```python
from build123d import *

# Parameters (mm, degrees)
ESQUISSE1_R             = 1.6
BOSS_EXTRU_1_DEPTH      = 3
ENL_V_MAT_EXTRU_1_DEPTH = 10


with BuildPart() as part:
    # Esquisse1 → Boss.-Extru.1 (new body)
    with BuildSketch(Plane.XY):
        Polygon((-13.474992457, 0.072428093), (-16.723236211, 3.320852512), (-154.236345188, 3.320852512), (-157.478985875, 0.078211825), (-157.478985875, -70.04068474), (-131.779420125, -114.771472067), (-127.355917516, -115.9649154), (-106.081983802, -103.720194839), (-66.092540926, -97.775797545), (-55.98795635, -83.933633781), (-16.581747648, -83.933633781), (-13.474992457, -80.826878591), align=None)
        Polygon((-126.111124489, -102.556497988), (-140.02282508, -78.342807898), (-141.407217303, -75.981121034), (-120.346626934, -63.796065222), (-120.346308835, -12.429484403), (-101.345774335, -12.429484403), (-101.345774335, -9.929307079), (-82.344426674, -9.929307079), (-82.344426674, -7.679926158), (-62.343149943, -7.681038584), (-62.343149943, -9.929307079), (-43.477687779, -9.929307079), (-43.477687779, -14.679643994), (-24.474992457, -14.679643994), (-24.474992457, -72.933633781), (-61.577157206, -72.933633781), (-72.263087593, -87.572177036), (-109.761976756, -93.1463556), align=None, mode=Mode.SUBTRACT)
        with Locations((-68.897334865, -93.137788223)):
            Circle(ESQUISSE1_R, mode=Mode.SUBTRACT)
        with Locations((-146.02282508, -1.677868186)):
            Circle(ESQUISSE1_R, mode=Mode.SUBTRACT)
        with Locations((-18.474992457, -1.68453516)):
            Circle(ESQUISSE1_R, mode=Mode.SUBTRACT)
    extrude(amount=BOSS_EXTRU_1_DEPTH)

    # Esquisse2 → Enlèv. mat.-Extru.1 (cut)
    with BuildSketch(Plane.XY.offset(3)):
        with BuildLine():
            Line((-25.386559375, 6.054162745), (-25.386559375, -4.679147488))
            ThreePointArc((-25.386559375, -4.679147488), (-26.386559375, -5.679147488), (-27.386559375, -4.679147488))
            Line((-27.386559375, -4.679147488), (-27.386559375, 6.054162745))
            ThreePointArc((-27.386559375, 6.054162745), (-26.386559375, 7.054162745), (-25.386559375, 6.054162745))
        make_face()
        with BuildLine():
            Line((-29.386559375, 6.054162745), (-29.386559375, -4.679147488))
            ThreePointArc((-29.386559375, -4.679147488), (-30.386559375, -5.679147488), (-31.386559375, -4.679147488))
            Line((-31.386559375, -4.679147488), (-31.386559375, 6.054162745))
            ThreePointArc((-31.386559375, 6.054162745), (-30.386559375, 7.054162745), (-29.386559375, 6.054162745))
        make_face()
        with BuildLine():
            Line((-33.386559375, 6.054162745), (-33.386559375, -4.679147488))
            ThreePointArc((-33.386559375, -4.679147488), (-34.386559375, -5.679147488), (-35.386559375, -4.679147488))
            Line((-35.386559375, -4.679147488), (-35.386559375, 6.054162745))
            ThreePointArc((-35.386559375, 6.054162745), (-34.386559375, 7.054162745), (-33.386559375, 6.054162745))
        make_face()
        with BuildLine():
            Line((-37.386559375, 6.054162745), (-37.386559375, -4.679147488))
            ThreePointArc((-37.386559375, -4.679147488), (-38.386559375, -5.679147488), (-39.386559375, -4.679147488))
            Line((-39.386559375, -4.679147488), (-39.386559375, 6.054162745))
            ThreePointArc((-39.386559375, 6.054162745), (-38.386559375, 7.054162745), (-37.386559375, 6.054162745))
        make_face()
        with BuildLine():
            Line((-41.386559375, 6.054162745), (-41.386559375, -4.679147488))
            ThreePointArc((-41.386559375, -4.679147488), (-42.386559375, -5.679147488), (-43.386559375, -4.679147488))
            Line((-43.386559375, -4.679147488), (-43.386559375, 6.054162745))
            ThreePointArc((-43.386559375, 6.054162745), (-42.386559375, 7.054162745), (-41.386559375, 6.054162745))
        make_face()
        with BuildLine():
            Line((-45.386559375, 6.054162745), (-45.386559375, -4.679147488))
            ThreePointArc((-45.386559375, -4.679147488), (-46.386559375, -5.679147488), (-47.386559375, -4.679147488))
            Line((-47.386559375, -4.679147488), (-47.386559375, 6.054162745))
            ThreePointArc((-47.386559375, 6.054162745), (-46.386559375, 7.054162745), (-45.386559375, 6.054162745))
        make_face()
        with BuildLine():
            Line((-49.386559375, 6.054162745), (-49.386559375, -4.679147488))
            ThreePointArc((-49.386559375, -4.679147488), (-50.386559375, -5.679147488), (-51.386559375, -4.679147488))
            Line((-51.386559375, -4.679147488), (-51.386559375, 6.054162745))
            ThreePointArc((-51.386559375, 6.054162745), (-50.386559375, 7.054162745), (-49.386559375, 6.054162745))
        make_face()
        with BuildLine():
            Line((-53.386559375, 6.054162745), (-53.386559375, -4.679147488))
            ThreePointArc((-53.386559375, -4.679147488), (-54.386559375, -5.679147488), (-55.386559375, -4.679147488))
            Line((-55.386559375, -4.679147488), (-55.386559375, 6.054162745))
            ThreePointArc((-55.386559375, 6.054162745), (-54.386559375, 7.054162745), (-53.386559375, 6.054162745))
        make_face()
        with BuildLine():
            Line((-57.386559375, 6.054162745), (-57.386559375, -4.679147488))
            ThreePointArc((-57.386559375, -4.679147488), (-58.386559375, -5.679147488), (-59.386559375, -4.679147488))
            Line((-59.386559375, -4.679147488), (-59.386559375, 6.054162745))
            ThreePointArc((-59.386559375, 6.054162745), (-58.386559375, 7.054162745), (-57.386559375, 6.054162745))
        make_face()
        with BuildLine():
            Line((-61.386559375, 6.054162745), (-61.386559375, -4.679147488))
            ThreePointArc((-61.386559375, -4.679147488), (-62.386559375, -5.679147488), (-63.386559375, -4.679147488))
            Line((-63.386559375, -4.679147488), (-63.386559375, 6.054162745))
            ThreePointArc((-63.386559375, 6.054162745), (-62.386559375, 7.054162745), (-61.386559375, 6.054162745))
        make_face()
        with BuildLine():
            Line((-65.386559375, 6.054162745), (-65.386559375, -4.679147488))
            ThreePointArc((-65.386559375, -4.679147488), (-66.386559375, -5.679147488), (-67.386559375, -4.679147488))
            Line((-67.386559375, -4.679147488), (-67.386559375, 6.054162745))
            ThreePointArc((-67.386559375, 6.054162745), (-66.386559375, 7.054162745), (-65.386559375, 6.054162745))
        make_face()
        with BuildLine():
            Line((-69.386559375, 6.054162745), (-69.386559375, -4.679147488))
            ThreePointArc((-69.386559375, -4.679147488), (-70.386559375, -5.679147488), (-71.386559375, -4.679147488))
            Line((-71.386559375, -4.679147488), (-71.386559375, 6.054162745))
            ThreePointArc((-71.386559375, 6.054162745), (-70.386559375, 7.054162745), (-69.386559375, 6.054162745))
        make_face()
        with BuildLine():
            Line((-73.386559375, 6.054162745), (-73.386559375, -4.679147488))
            ThreePointArc((-73.386559375, -4.679147488), (-74.386559375, -5.679147488), (-75.386559375, -4.679147488))
            Line((-75.386559375, -4.679147488), (-75.386559375, 6.054162745))
            ThreePointArc((-75.386559375, 6.054162745), (-74.386559375, 7.054162745), (-73.386559375, 6.054162745))
        make_face()
        with BuildLine():
            Line((-77.386559375, 6.054162745), (-77.386559375, -4.679147488))
            ThreePointArc((-77.386559375, -4.679147488), (-78.386559375, -5.679147488), (-79.386559375, -4.679147488))
            Line((-79.386559375, -4.679147488), (-79.386559375, 6.054162745))
            ThreePointArc((-79.386559375, 6.054162745), (-78.386559375, 7.054162745), (-77.386559375, 6.054162745))
        make_face()
        with BuildLine():
            Line((-81.386559375, 6.054162745), (-81.386559375, -4.679147488))
            ThreePointArc((-81.386559375, -4.679147488), (-82.386559375, -5.679147488), (-83.386559375, -4.679147488))
            Line((-83.386559375, -4.679147488), (-83.386559375, 6.054162745))
            ThreePointArc((-83.386559375, 6.054162745), (-82.386559375, 7.054162745), (-81.386559375, 6.054162745))
        make_face()
        with BuildLine():
            Line((-85.386559375, 6.054162745), (-85.386559375, -4.679147488))
            ThreePointArc((-85.386559375, -4.679147488), (-86.386559375, -5.679147488), (-87.386559375, -4.679147488))
            Line((-87.386559375, -4.679147488), (-87.386559375, 6.054162745))
            ThreePointArc((-87.386559375, 6.054162745), (-86.386559375, 7.054162745), (-85.386559375, 6.054162745))
        make_face()
        with BuildLine():
            Line((-89.386559375, 6.054162745), (-89.386559375, -4.679147488))
            ThreePointArc((-89.386559375, -4.679147488), (-90.386559375, -5.679147488), (-91.386559375, -4.679147488))
            Line((-91.386559375, -4.679147488), (-91.386559375, 6.054162745))
            ThreePointArc((-91.386559375, 6.054162745), (-90.386559375, 7.054162745), (-89.386559375, 6.054162745))
        make_face()
        with BuildLine():
            Line((-93.386559375, 6.054162745), (-93.386559375, -4.679147488))
            ThreePointArc((-93.386559375, -4.679147488), (-94.386559375, -5.679147488), (-95.386559375, -4.679147488))
            Line((-95.386559375, -4.679147488), (-95.386559375, 6.054162745))
            ThreePointArc((-95.386559375, 6.054162745), (-94.386559375, 7.054162745), (-93.386559375, 6.054162745))
        make_face()
        with BuildLine():
            Line((-97.386559375, 6.054162745), (-97.386559375, -4.679147488))
            ThreePointArc((-97.386559375, -4.679147488), (-98.386559375, -5.679147488), (-99.386559375, -4.679147488))
            Line((-99.386559375, -4.679147488), (-99.386559375, 6.054162745))
            ThreePointArc((-99.386559375, 6.054162745), (-98.386559375, 7.054162745), (-97.386559375, 6.054162745))
        make_face()
        with BuildLine():
            Line((-101.386559375, 6.054162745), (-101.386559375, -4.679147488))
            ThreePointArc((-101.386559375, -4.679147488), (-102.386559375, -5.679147488), (-103.386559375, -4.679147488))
            Line((-103.386559375, -4.679147488), (-103.386559375, 6.054162745))
            ThreePointArc((-103.386559375, 6.054162745), (-102.386559375, 7.054162745), (-101.386559375, 6.054162745))
        make_face()
    extrude(amount=-ENL_V_MAT_EXTRU_1_DEPTH, mode=Mode.SUBTRACT)


solid = part.part
```
Build history of the part. All positions in model axes, mm. A direction names the side the tool comes from. Give positions to 0.01 mm unless a question says otherwise; leave off trailing zeros. Order: outer loops, then holes, each group sorted by start corner. A loop starts at its lowest first (then second) coordinate and runs counter-clockwise, first axis right, second up. Notation, with made-up numbers: M 47,17.5 L 82,17.5 A25 cw 82,42.5 Z; hole C 45.5,0 d8. An arc over 180 degrees is marked long. Return JSON: item names as keys, results as strings.
Q1. Two-plate mould, pull along X, no slides. Class faces 4 (the face through (-144.81, -92.09, 1.48)), 5 (the face through (-61.387, -1, 2)), 6 (the face through (-15.05, -82.4, 1.48)), 7 (the face through (-128, 3.321, 1)): pulls with the +X half, pulls with the -X half, needs draft (parallel to the pull), parting line crosses it, or undercut.
Answer list:
{"face 4": "pulls with the -X half", "face 5": "undercut", "face 6": "pulls with the +X half", "face 7": "needs draft"}
Q2. 3-axis set-ups, long thin cutter, end or side, ignore diameter. For faces 1 (the face through (-86.37, -100.79, 1.48)), 2 (the face through (-81.387, -1, 2)), 3 (the face through (-43.478, -12, 1)): which of +Z, -Z, +X, -X, +Y, -Y reach the whole face in a straight line?
Answer list:
{"face 1": "+Z, -Z, +X, -Y", "face 2": "+Z, -Z, +Y", "face 3": "+Z, -Z"}
Q3. Band-saw the part on C-C (y = -85.5). Give the cut face in (x, z), then the cut area to 3 significant figures.
Answer list:
{"outline": "M -148.6,0 L -135.91,0 L -135.91,3 L -148.6,3 Z; M -70.75,0 L -57.13,0 L -57.13,3 L -70.75,3 Z", "area": "78.9 mm^2"}
Q4. Flat gauge pins, fed straight in: pin 1 (0.9 mm diameter, centred on y = 1.5, z = 1, fed in from +X); pin 2 (1.5 mm diameter, centred on y = -96, z = 1, fed in from +X); pin 3 (3.5 mm diameter, centred on x = -146.02, y = -1.68, fed in from -Z); pin 4 (1.5 mm diameter, centred on y = -101.5, z = 2, fed in from -X). Where does each tip first touch, or does it go through?
Answer list:
{"pin 1": "stops at x = -14.45", "pin 2": "stops at x = -64.25", "pin 3": "stops at z = 0", "pin 4": "stops at x = -139.84"}
Q5. Wall check: probe 1 along X at (y, z) = (-12, 0.85) (3 decimals); probe 2 along X at (y, z) = (-33, 2.05) (3 decimals); probe 3 along Y at (x, z) = (-52, 1.7). Give the ranges that are in metal, low to high. Write a range as from..to.
Answer list:
{"probe 1": "x = -157.479..-101.346, -43.478..-13.475", "probe 2": "x = -157.479..-120.346, -24.475..-13.475", "probe 3": "y = -83.93..-72.93, -9.93..3.32"}
Q6. Band-saw the part on A-A (y = -42.5). Give the cut face in (x, z) (1 decimal), then the cut area to 3 significant figures.
Answer list:
{"outline": "M -157.5,0 L -120.3,0 L -120.3,3 L -157.5,3 Z; M -24.5,0 L -13.5,0 L -13.5,3 L -24.5,3 Z", "area": "144 mm^2"}
Q7. Band-saw the part on B-B (z = 0.9). Count the separate pieces of the cut face and the enclosed holes in it, then the cut area to 3 significant figures.
Answer list:
{"separate pieces": "1", "enclosed holes": "4", "area": "6,420 mm^2"}
